Autodesk Inventor part; units mm, degrees
ref_plane "YZ Plane" through (0, 0, 0) normal (1, 0, 0) x (0, 1, 0)
ref_plane "XZ Plane" through (0, 0, 0) normal (0, 1, 0) x (-1, 0, 0)
ref_plane "XY Plane" through (0, 0, 0) normal (0, 0, 1) x (1, 0, 0)
sketch "Sketch1" plane through (0, 0, 0) normal (0, 0, 1) x (1, 0, 0)
  line L0 (0, 0) -> (50.8, 0)
  line L1 (50.8, 0) -> (50.8, 6.35)
  line L2 (50.8, 6.35) -> (0, 6.35)
  line L3 (0, 6.35) -> (0, 0)
  circle A0 centre (3.175, 3.175) radius 1.5875
  circle A1 centre (15.875, 3.175) radius 1.5875
  line L4 (41.275, 1.5875) -> (47.625, 1.5875)
  line L5 (47.625, 1.5875) -> (47.625, 4.5085)
  line L6 (47.625, 4.5085) -> (41.275, 4.5085)
  line L7 (41.275, 4.5085) -> (41.275, 1.5875)
  dimension "d0" = 50.8
  dimension "d1" = 6.35
  dimension "d2" = 3.175
  dimension "d3" = 3.175
  dimension "d4" = 3.175
  dimension "d5" = 3.175
  dimension "d6" = 3.175
  dimension "d7" = 12.7
  dimension "d8" = 2.921
  dimension "d9" = 1.5875
  dimension "d10" = 6.35
  dimension "d11" = 3.175
extrude "Extrusion1" add sketch "Sketch1" along normal blind 3.175
chamfer "Chamfer1" distance 1.5875 angle 45 2 edges at (0, 6.35, 1.5875) (0, 0, 1.5875)
properties part number "camera_arm"
Source: CAD feature listing. Evaluate the final solid. Frame: model axes, mm. A direction names the side the tool comes from. Give positions to 0.01 mm unless a question says otherwise; leave off trailing zeros. Write each loop counter-clockwise with the first axis right and the second up, starting at its lowest first coordinate (ties: lowest second). Pieces come first, ordered by that corner, then holes. Notation, with made-up numbers: (36, 19) -> (55, 19) arc R21 ccw to (55, 52) -> close; hole circle Ø10 at (36, -21). An arc over 180 degrees is marked (long way). Return JSON: item names as keys, results as strings. Group by question number.
1. Mould query, pull axis X, two halves, no side actions, for faces 1 (the face through (26, 0, 2)), 2 (the face through (50.8, 3, 2)), 3 (the face through (44, 4.508, 2)). Classes: +X half, -X half, draft (parallel to the pull), parting line (faces both ways), or undercut.
2. Access query for faces 4 (the face through (25, 3, 3.175)), 5 (the face through (41.275, 3, 2)). Directions: +Z, -Z, +X, -X, +Y, -Y. A direction counts if a zero-diameter tool reaches every point of the face in a straight line with its end or side. Return the directions, or none.
3. Pin query (flat end, axial travel): pin 1 Ø1.9 at (x, y) = (15.875, 3.175) entering from +Z. Return the tip coordinate at first contact, or that it passes through.
4. Material intervals for line 1 (X direction, y = 3.25, z = 1.05) (3 decimals); line 2 (X direction, y = 3.5, z = 2.8) (3 decimals); line 3 (Y direction, x = 43.5, z = 1.85), sorted ascending. Write a range as from..to.
5. Section B-B, the plane x = 3.5. Output: boundary loops of the cut face in (y, z) (3 decimals).
6. Section A-A, the plane z = 1.6. Count the separate pieces of the cut face and the enclosed holes in it, then the cut area to 3 significant figures.
Determined:
{
 "1": {"face 1": "draft", "face 2": "+X half", "face 3": "undercut"},
 "2": {"face 4": "+Z, +X, -X, +Y, -Y", "face 5": "+Z, -Z"},
 "3": {"pin 1": "passes through"},
 "4": {"line 1": "x = 0..1.589, 4.761..14.289, 17.461..41.275, 47.625..50.8", "line 2": "x = 0..1.621, 4.729..14.321, 17.429..41.275, 47.625..50.8", "line 3": "y = 0..1.59, 4.51..6.35"},
 "5": {"outline": "(0, 0) -> (1.621, 0) -> (1.621, 3.175) -> (0, 3.175) -> close; (4.729, 0) -> (6.35, 0) -> (6.35, 3.175) -> (4.729, 3.175) -> close"},
 "6": {"separate pieces": "1", "enclosed holes": "3", "area": "286 mm2"}
}
